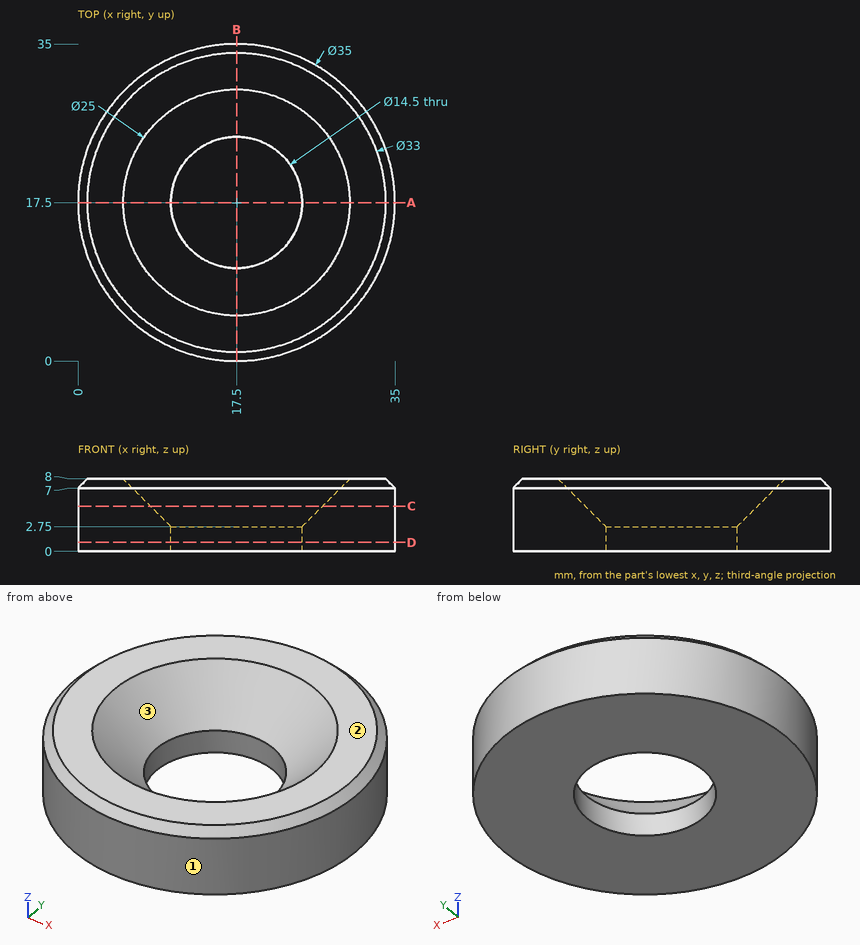
Answer from the drawing. Dimensions are ordinates in mm from the lowest x, y and z of the part. Round coordinates to 2 decimals unless told otherwise and drop trailing zeros. Write each loop counter-clockwise with the first axis right and the second up, starting at its lowest first coordinate (ties: lowest second). Pieces come first, ordered by that corner, then holes.
1. Given pin 1 Ø2 at (y, z) = (19, 2.5) entering from -X; pin 2 Ø19 at (x, y) = (17.5, 17.5) entering from +Z; pin 3 Ø2 at (y, z) = (13, 5) entering from +X, each flat-ended and moving along its own axis, determine where each tip first touches the part or whether it passes through.
2. Straight lines are drawn through the part: L1, parallel to Y at x = 17.5, z = 1.15; L2, parallel to Y at x = 23.5, z = 4; L3, parallel to X at y = 15, z = 5.75. For each, find the intervals that lie inside material, in ascending order.
3. The part is cut by section A-A, the plane y = 17.5. Determine the outline of the cut face in (x, z).
4. The part is cut by section D-D, the plane z = 1. Determine the outline of the cut face in (x, y), then the cut area to 3 significant figures.
5. The part is cut by section C-C, the plane z = 5. Determine the outline of the cut face in (x, y).
6. Determine the mould class of the marked faces 1, 2 and 3 for opening direction X: pulls with the +X half, pulls with the -X half, needs draft (parallel to the pull), parting line crosses it, or undercut.
Values:
1. pin 1: stops at x = 0.01
1. pin 2: stops at z = 5
1. pin 3: stops at x = 34.65
2. L1: y = 0 to 10.25, 24.75 to 35
2. L2: y = 1.06 to 11.48, 23.52 to 33.94
2. L3: x = 0.18 to 7.56, 27.44 to 34.82
3. outline: (0, 0) - (10.25, 0) - (10.25, 2.75) - (5, 8) - (1, 8) - (0, 7) - close; (24.75, 0) - (35, 0) - (35, 7) - (34, 8) - (30, 8) - (24.75, 2.75) - close
4. outline: circle Ø35 at (17.5, 17.5); hole circle Ø14.5 at (17.5, 17.5)
4. area: 797 mm2
5. outline: circle Ø35 at (17.5, 17.5); hole circle Ø19 at (17.5, 17.5)
6. face 1: parting line crosses it
6. face 2: needs draft
6. face 3: undercut
